```python
from build123d import *

# Parameters (mm, degrees)
SKETCH1_R             = 3.175
BOSS_EXTRUDE1_DEPTH   = 3.175
FILLET1_R             = 3.175
F_2_CLEARANCE_HOLE1_D = 2.7051
F_2_CLEARANCE_HOLE2_D = 2.7051
CUT_EXTRUDE1_DEPTH    = 131.094336971


with BuildPart() as part:
    # Sketch1 → Boss-Extrude1 (new body)
    with BuildSketch(Plane.XY):
        with BuildLine():
            ThreePointArc((-89.910569383, 80.265306107), (-93.701723521, 77.150666629), (-96.021422346, 81.474186739))
            Line((-96.021422346, 81.474186739), (-99.521422346, 72.974186739))
            ThreePointArc((-99.521422346, 72.974186739), (-95.969415245, 74.879945585), (-93.410569383, 71.765306107))
            ThreePointArc((-93.410569383, 71.765306107), (-94.340505353, 69.520242077), (-96.585569383, 68.590306107))
            Line((-96.585569383, 68.590306107), (-49.585569383, 68.590306107))
            ThreePointArc((-49.585569383, 68.590306107), (-52.223638848, 73.532002034), (-46.649716421, 72.974186739))
            Line((-46.649716421, 72.974186739), (-50.149716421, 81.474186739))
            ThreePointArc((-50.149716421, 81.474186739), (-49.970929905, 80.881460245), (-49.910569383, 80.265306107))
            ThreePointArc((-49.910569383, 80.265306107), (-55.330633414, 78.020242077), (-53.085569383, 83.440306107))
            Line((-53.085569383, 83.440306107), (-93.085569383, 83.440306107))
            ThreePointArc((-93.085569383, 83.440306107), (-90.840505353, 82.510370138), (-89.910569383, 80.265306107))
        make_face()
        with Locations((-93.085569383, 80.265306107)):
            Circle(SKETCH1_R)
        with Locations((-96.585569383, 71.765306107)):
            Circle(SKETCH1_R)
        with Locations((-49.585569383, 71.765306107)):
            Circle(SKETCH1_R)
        with Locations((-53.085569383, 80.265306107)):
            Circle(SKETCH1_R)
        with BuildLine():
            ThreePointArc((-46.410569383, 71.765306107), (-47.340505353, 69.520242077), (-49.585569383, 68.590306107))
            Line((-49.585569383, 68.590306107), (-49.585569383, 51.940306107))
            ThreePointArc((-49.585569383, 51.940306107), (-47.340505353, 51.010370138), (-46.410569383, 48.765306107))
            Line((-46.410569383, 48.765306107), (-46.410569383, 71.765306107))
        make_face()
        with Locations((-49.585569383, 48.765306107)):
            Circle(SKETCH1_R)
        with Locations((-53.085569383, 40.265306107)):
            Circle(SKETCH1_R)
        with BuildLine():
            Line((-49.585569383, 51.940306107), (-96.585569383, 51.940306107))
            ThreePointArc((-96.585569383, 51.940306107), (-94.340505353, 51.010370138), (-93.410569383, 48.765306107))
            ThreePointArc((-93.410569383, 48.765306107), (-95.969415245, 45.650666629), (-99.521422346, 47.556425476))
            Line((-99.521422346, 47.556425476), (-96.021422346, 39.056425476))
            ThreePointArc((-96.021422346, 39.056425476), (-93.701723521, 43.379945585), (-89.910569383, 40.265306107))
            ThreePointArc((-89.910569383, 40.265306107), (-90.840505353, 38.020242077), (-93.085569383, 37.090306107))
            Line((-93.085569383, 37.090306107), (-53.085569383, 37.090306107))
            ThreePointArc((-53.085569383, 37.090306107), (-55.330633414, 42.510370138), (-49.910569383, 40.265306107))
            ThreePointArc((-49.910569383, 40.265306107), (-49.970929905, 39.649151969), (-50.149716421, 39.056425476))
            Line((-50.149716421, 39.056425476), (-46.649716421, 47.556425476))
            ThreePointArc((-46.649716421, 47.556425476), (-52.223638848, 46.998610181), (-49.585569383, 51.940306107))
        make_face()
        with Locations((-93.085569383, 40.265306107)):
            Circle(SKETCH1_R)
        with Locations((-96.585569383, 48.765306107)):
            Circle(SKETCH1_R)
        with BuildLine():
            ThreePointArc((-96.585569383, 68.590306107), (-98.830633414, 69.520242077), (-99.760569383, 71.765306107))
            Line((-99.760569383, 71.765306107), (-99.760569383, 48.765306107))
            ThreePointArc((-99.760569383, 48.765306107), (-98.830633414, 51.010370138), (-96.585569383, 51.940306107))
            Line((-96.585569383, 51.940306107), (-96.585569383, 68.590306107))
        make_face()
    extrude(amount=BOSS_EXTRUDE1_DEPTH)

    # Fillet1
    fillet1_edges = [part.edges().sort_by_distance(p)[0] for p in [
        (-96.585569383, 68.590306107, 1.5875),
        (-96.585569383, 51.940306107, 1.5875),
        (-49.585569383, 51.940306107, 1.5875),
        (-49.585569383, 68.590306107, 1.5875),
    ]]
    fillet(fillet1_edges, radius=FILLET1_R)

    # #2 Clearance Hole1 (through all)
    with Locations(Plane.XY.offset(3.175)):
        with Locations((-93.085569383, 80.265306107), (-53.085569383, 80.265306107), (-53.085569383, 40.265306107), (-93.085569383, 40.265306107)):
            Hole(F_2_CLEARANCE_HOLE1_D / 2)

    # #2 Clearance Hole2 (through all)
    with Locations(Plane.XY.offset(3.175)):
        with Locations((-96.585569383, 71.765306107), (-49.585569383, 71.765306107), (-49.585569383, 48.765306107), (-96.585569383, 48.765306107)):
            Hole(F_2_CLEARANCE_HOLE2_D / 2)

    # Sketch6 → Cut-Extrude1 (cut, through all)
    with BuildSketch(Plane.XY.offset(3.175)):
        with BuildLine():
            Line((-84.198069383, 80.265306107), (-61.973069383, 80.265306107))
            ThreePointArc((-61.973069383, 80.265306107), (-57.723069383, 76.015306107), (-61.973069383, 71.765306107))
            Line((-61.973069383, 71.765306107), (-84.198069383, 71.765306107))
            ThreePointArc((-84.198069383, 71.765306107), (-88.448069383, 76.015306107), (-84.198069383, 80.265306107))
        make_face()
        with BuildLine():
            Line((-84.198069383, 40.265306107), (-61.973069383, 40.265306107))
            ThreePointArc((-61.973069383, 40.265306107), (-57.723069383, 44.515306107), (-61.973069383, 48.765306107))
            Line((-61.973069383, 48.765306107), (-84.198069383, 48.765306107))
            ThreePointArc((-84.198069383, 48.765306107), (-88.448069383, 44.515306107), (-84.198069383, 40.265306107))
        make_face()
    extrude(amount=-CUT_EXTRUDE1_DEPTH, mode=Mode.SUBTRACT)


solid = part.part
```
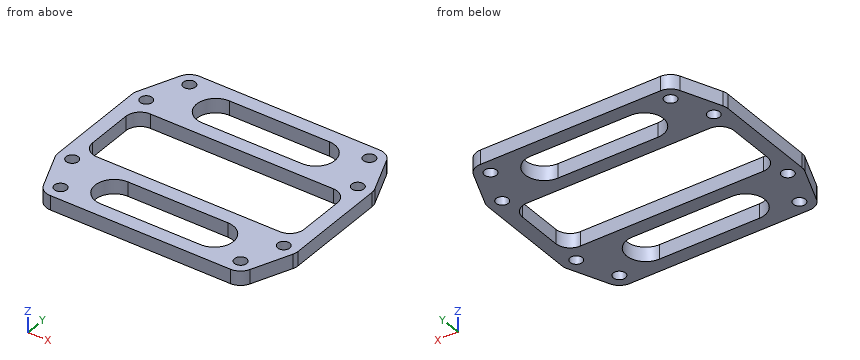
Check sheet for the modelled part. Datum: model origin and axes. Units: mm. Give positions to 0.01 mm unless a question says otherwise; leave off trailing zeros. Order: outer loops, then holes, each group sorted by start corner. A loop starts at its lowest first (then second) coordinate and runs counter-clockwise, first axis right, second up. Notation, with made-up numbers: M -30,-36.5 L 27,-36.5 A30 ccw 27,2.5 Z; hole C 33,35 d11. An arc over 180 degrees is marked long. Answer in a Markdown table with one row per item. Add a question column.
Q1. Sectioned sample at B-B, the plane x = -57. Record the boundary of the cut face in (y, z) (3 decimals).
Q2. Sectioned sample at C-C, the plane y = 71. Record the boundary of the cut face in (x, z) (3 decimals), and give its area (3 significant figures).
Q3. Sectioned sample at D-D, the plane x = -76. Record the boundary of the cut face in (y, z) (3 decimals).
Q4. Gauge pin test, flat ends, axial feed: pin 1 Ø2 at (x, y) = (-93.09, 80.27) entering from -Z; pin 2 Ø3.5 at (x, y) = (-49.59, 48.77) entering from -Z. Record the tip position at first contact, or that the pin passes through.
Q5. Sectioned sample at A-A, the plane y = 59. Record the boundary of the cut face in (x, z) (3 decimals).
Q6. Thickness scan on L1, parallel to Y at x = -78, z = 0.3; L2, parallel to Y at x = -53, z = 2.7; L3, parallel to X at y = 63, z = 2.35. Record the ranges inside material, lowest first.
Verdict:
| question | item | result |
|---|---|---|
| 1 | outline | M 37.09,0 L 51.94,0 L 51.94,3.175 L 37.09,3.175 Z; M 68.59,0 L 83.44,0 L 83.44,3.175 L 68.59,3.175 Z |
| 2 | outline | M -99.761,0 L -97.701,0 L -97.701,3.175 L -99.761,3.175 Z; M -95.47,0 L -50.701,0 L -50.701,3.175 L -95.47,3.175 Z; M -48.47,0 L -46.411,0 L -46.411,3.175 L -48.47,3.175 Z |
| 2 | area | 155 mm² |
| 3 | outline | M 37.09,0 L 40.265,0 L 40.265,3.175 L 37.09,3.175 Z; M 48.765,0 L 51.94,0 L 51.94,3.175 L 48.765,3.175 Z; M 68.59,0 L 71.765,0 L 71.765,3.175 L 68.59,3.175 Z; M 80.265,0 L 83.44,0 L 83.44,3.175 L 80.265,3.175 Z |
| 4 | pin 1 | through |
| 4 | pin 2 | z = 0 |
| 5 | outline | M -99.761,0 L -96.586,0 L -96.586,3.175 L -99.761,3.175 Z; M -49.586,0 L -46.411,0 L -46.411,3.175 L -49.586,3.175 Z |
| 6 | L1 | 37.09 to 40.27, 48.77 to 51.94, 68.59 to 71.77, 80.27 to 83.44 |
| 6 | L2 | 37.09 to 38.92, 41.62 to 51.94, 68.59 to 78.92, 81.62 to 83.44 |
| 6 | L3 | -99.76 to -96.59, -49.59 to -46.41 |
